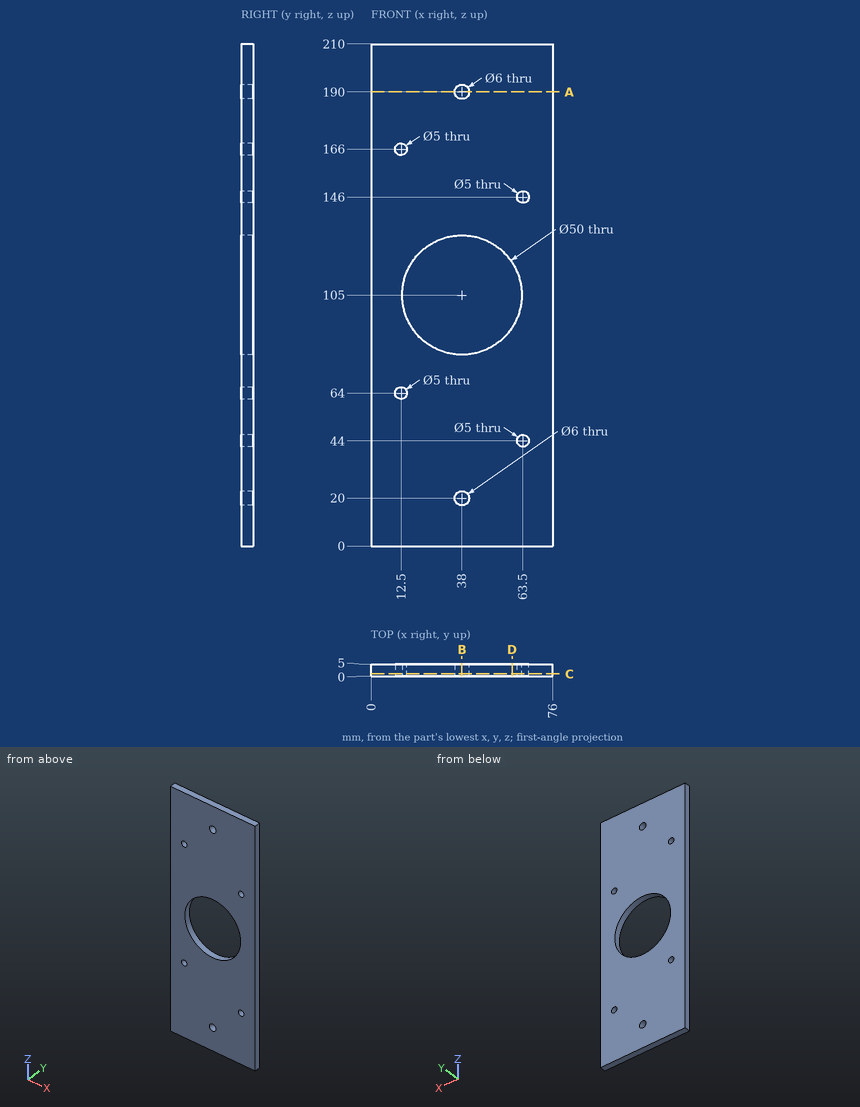
Check sheet for the drawn part. Datum: minimum x, y, z corner. Units: mm. Give positions to 0.01 mm unless a question says otherwise; leave off trailing zeros. Order: outer loops, then holes, each group sorted by start corner. A loop starts at its lowest first (then second) coordinate and runs counter-clockwise, first axis right, second up. Notation, with made-up numbers: (-35.5, 83.25) -> (8.5, 83.25) arc R20 cw to (8.5, 91.25) -> close; hole circle Ø6 at (60, 38.5). An arc over 180 degrees is marked (long way). Return JSON: item names as keys, results as strings.
1. Cross-section at A-A, the plane z = 190. Record the cut outline in (x, y), plus the area to 3 significant figures.
From the geometry:
{"outline": "(0, 0) -> (35, 0) -> (35, 5) -> (0, 5) -> close; (41, 0) -> (76, 0) -> (76, 5) -> (41, 5) -> close", "area": "350 mm^2"}
2. Cross-section at B-B, the plane x = 38. Record the cut outline in (y, z), plus the area to 3 significant figures.
From the geometry:
{"outline": "(0, 0) -> (5, 0) -> (5, 17) -> (0, 17) -> close; (0, 23) -> (5, 23) -> (5, 80) -> (0, 80) -> close; (0, 130) -> (5, 130) -> (5, 187) -> (0, 187) -> close; (0, 193) -> (5, 193) -> (5, 210) -> (0, 210) -> close", "area": "740 mm^2"}
3. Cross-section at D-D, the plane x = 59. Record the cut outline in (y, z).
From the geometry:
{"outline": "(0, 0) -> (5, 0) -> (5, 91.44) -> (0, 91.44) -> close; (0, 118.56) -> (5, 118.56) -> (5, 210) -> (0, 210) -> close"}
4. Material ranges on probe 1 along Z at (x, y) = (12.5, 3.3); probe 2 along Z at (x, y) = (38, 3.45); probe 3 along X at (y, z) = (1.3, 166), recorded low to high. Write a range as [from, to].
From the geometry:
{"probe 1": "[0, 61.5], [66.5, 163.5], [168.5, 210]", "probe 2": "[0, 17], [23, 80], [130, 187], [193, 210]", "probe 3": "[0, 10], [15, 76]"}
5. Cross-section at C-C, the plane y = 0.9. Record the cut outline in (x, z).
From the geometry:
{"outline": "(0, 0) -> (76, 0) -> (76, 210) -> (0, 210) -> close; hole circle Ø5 at (12.5, 64); hole circle Ø5 at (12.5, 166); hole circle Ø50 at (38, 105); hole circle Ø6 at (38, 20); hole circle Ø6 at (38, 190); hole circle Ø5 at (63.5, 44); hole circle Ø5 at (63.5, 146)"}
